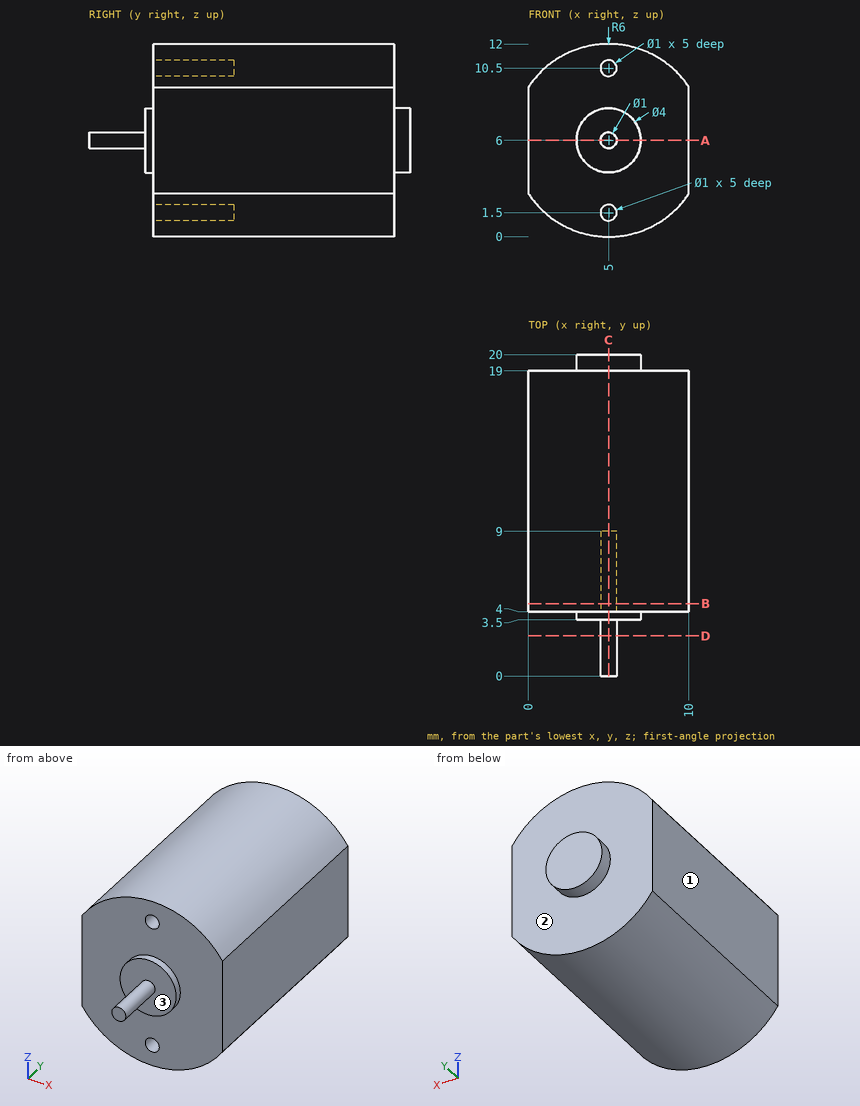
Geometry: see drawing. Coordinates: mm, zero at the bounding-box minimum. A direction names the side the tool comes from. Give positions to 0.01 mm unless a question says otherwise; leave off trailing zeros. Loops run counter-clockwise (first coordinate to the right, second up) from the corner with the lowest first, then second, coordinate; pieces in that order, holes last. Notation, with made-up numbers: M -39,61 L 7,61 A23 cw 7,70 Z; hole C -0.75,34 d10. An arc over 180 degrees is marked long. Use one line per item in the form item = value.
1. Section query D-D, the plane y = 2.5. Return the cut outline in (x, z), and give its area (3 significant figures).
Numbers:
outline = C 5,6 d1
area = 0.785 mm²
2. Section query A-A, the plane z = 6. Return the cut outline in (x, y), and give its area (4 significant figures).
Numbers:
outline = M 0,4 L 3,4 L 3,3.5 L 4.5,3.5 L 4.5,0 L 5.5,0 L 5.5,3.5 L 7,3.5 L 7,4 L 10,4 L 10,19 L 7,19 L 7,20 L 3,20 L 3,19 L 0,19 Z
area = 159.5 mm²
3. Section query B-B, the plane y = 4.5. Return the cut outline in (x, z).
Numbers:
outline = M 0,2.68 A6 ccw 10,2.68 L 10,9.32 A6 ccw 0,9.32 Z; hole C 5,1.5 d1; hole C 5,10.5 d1
4. Line query: L1, parallel to Z at x = 5.25, y = 9.5; L2, parallel to Y at x = 6.5, z = 3.25; L3, parallel to Y at x = 5, z = 7.25. Output: solid intervals per line, ascending.
Numbers:
L1 = 0.01 to 11.99
L2 = 4 to 19
L3 = 3.5 to 20
5. Reachability of the marked faces 1, 2 and 3 from +Z, -Z, +X, -X, +Y, -Y: full face, straight path, thin tool, end or side. Return the list, or none.
Numbers:
face_1 = +Z, -Z, -X, +Y, -Y
face_2 = +Y
face_3 = -Y
6. Section query C-C, the plane x = 5. Return the cut outline in (y, z), and give its area (4 significant figures).
Numbers:
outline = M 0,5.5 L 3.5,5.5 L 3.5,4 L 4,4 L 4,2 L 9,2 L 9,1 L 4,1 L 4,0 L 19,0 L 19,4 L 20,4 L 20,8 L 19,8 L 19,12 L 4,12 L 4,11 L 9,11 L 9,10 L 4,10 L 4,8 L 3.5,8 L 3.5,6.5 L 0,6.5 Z
area = 179.5 mm²
7. First-contact query: pin 1 (2 mm diameter, centred on x = 3, z = 3.5, fed in from +Y); pin 2 (3 mm diameter, centred on x = 4.5, z = 7, fed in from -Y); pin 3 (0.5 mm diameter, centred on x = 5, z = 10.5, fed in from -Y). Flat tips, straight axial feed; report the tip coordinate or a pass-through.
Numbers:
pin_1 = 19
pin_2 = 0
pin_3 = 9
